```python
from build123d import *

# Parameters (mm, degrees)
LINEAR_AUSTRAGEN1_DEPTH      = 31.8
SKIZZE2_W                    = 3
SKIZZE2_H                    = 2
LINEAR_AUSTRAGEN2_DEPTH      = 2
SKIZZE4_W                    = 150
SKIZZE4_H                    = 1.45
LINEAR_START                 = -18
LINEAR_AUSTRAGEN3_DEPTH      = 18
LINEAR_AUSTRAGEN4_DEPTH      = 18
LINEAR_AUSTRAGEN5_DEPTH      = 0.5
LINEAR_AUSTRAGEN5_DEPTH_BACK = 0.5
SKIZZE8_W                    = 1
SKIZZE8_H                    = 2
LINEAR_AUSTRAGEN6_DEPTH      = 2.6
LINEAR_START_2               = -2.1
LINEAR_AUSTRAGEN7_DEPTH      = 2.1


with BuildPart() as part:
    # Skizze1 → Linear austragen1 (new body)
    with BuildSketch(Plane.XY):
        with BuildLine():
            Line((-2.5, -2.1), (2.5, -2.1))
            Line((2.5, -2.1), (2.5, 2))
            ThreePointArc((2.5, 2), (0, 2.5), (-2.5, 2))
            Line((-2.5, 2), (-2.5, -2.1))
        make_face()
    extrude(amount=LINEAR_AUSTRAGEN1_DEPTH)

    # Skizze2 → Rotation1 (revolve)
    with BuildSketch(Plane(origin=(0, 0, 0), x_dir=(0, 0, -1), z_dir=(1, 0, 0)), mode=Mode.PRIVATE) as rotation1_sk:
        with Locations((1.5, 1)):
            Rectangle(SKIZZE2_W, SKIZZE2_H)
    revolve(rotation1_sk.sketch.rotate(Axis((0, 0, -3), (0, 0, 1)), 270), axis=Axis((0, 0, -3), (0, 0, 1)))

    # Skizze3 → Linear austragen2 (add)
    with BuildSketch(Plane(origin=(0, 2.6, 0), x_dir=(-1, 0, 0), z_dir=(0, 1, 0))):
        Polygon((2.5, 23.05), (0.2, 23.05), (0.2, 24.35), (-0.2, 24.35), (-0.2, 23.05), (-2.5, 23.05), (-2.5, 22.65), (-0.2, 22.65), (-0.2, 21.35), (0.2, 21.35), (0.2, 22.65), (2.5, 22.65), align=None)
    extrude(amount=-LINEAR_AUSTRAGEN2_DEPTH)

    # Skizze4 → Rotation2 (revolve)
    with BuildSketch(Plane(origin=(0, 0, 0), x_dir=(0, 0, -1), z_dir=(1, 0, 0)), mode=Mode.PRIVATE) as rotation2_sk:
        with Locations((78, 0.725)):
            Rectangle(SKIZZE4_W, SKIZZE4_H)
    revolve(rotation2_sk.sketch.rotate(Axis((0, 0, -153), (0, 0, 1)), 270), axis=Axis((0, 0, -153), (0, 0, 1)))

    # Skizze5 → Linear austragen3 (add)
    with BuildSketch(Plane.XY.offset(-8).offset(LINEAR_START)):
        with BuildLine():
            Line((-2.95, 2.95), (-2.95, -1.95))
            Line((-2.95, -1.95), (-1.95, -2.95))
            Line((-1.95, -2.95), (1.95, -2.95))
            Line((1.95, -2.95), (2.95, -1.95))
            Line((2.95, -1.95), (2.95, 2.95))
            Line((2.95, 2.95), (1.95, 2.95))
            Line((1.95, 2.95), (1.320214964, 0.599610248))
            ThreePointArc((1.320214964, 0.599610248), (0, -1.45), (-1.320214964, 0.599610248))
            Line((-1.320214964, 0.599610248), (-1.95, 2.95))
            Line((-1.95, 2.95), (-2.95, 2.95))
        make_face()
    extrude(amount=LINEAR_AUSTRAGEN3_DEPTH)

    # Skizze6 → Linear austragen4 (add)
    with BuildSketch(Plane.XY.offset(-148)):
        with BuildLine():
            Line((-2.95, 2.95), (-2.95, -1.95))
            Line((-2.95, -1.95), (-1.95, -2.95))
            Line((-1.95, -2.95), (1.95, -2.95))
            Line((1.95, -2.95), (2.95, -1.95))
            Line((2.95, -1.95), (2.95, 2.95))
            Line((2.95, 2.95), (1.95, 2.95))
            Line((1.95, 2.95), (1.320214964, 0.599610248))
            ThreePointArc((1.320214964, 0.599610248), (0, -1.45), (-1.320214964, 0.599610248))
            Line((-1.320214964, 0.599610248), (-1.95, 2.95))
            Line((-1.95, 2.95), (-2.95, 2.95))
        make_face()
    extrude(amount=LINEAR_AUSTRAGEN4_DEPTH)

    # Skizze7 → Rotation3 (revolve)
    with BuildSketch(Plane(origin=(0, 0, 0), x_dir=(0, 0, -1), z_dir=(1, 0, 0)), mode=Mode.PRIVATE) as rotation3_sk:
        with BuildLine():
            Line((153, 0), (153, 2.5))
            Line((153, 2.5), (153.5, 3))
            Line((153.5, 3), (154, 3))
            ThreePointArc((154, 3), (154.75, 2.799038106), (155.5, 3))
            Line((155.5, 3), (156, 3))
            ThreePointArc((156, 3), (156.5, 2.866025404), (157, 3))
            Line((157, 3), (162.82871818, 3))
            Line((162.82871818, 3), (168.5, 4))
            Line((168.5, 4), (178.5, 4))
            Line((178.5, 4), (178.5, 3.5))
            Line((178.5, 3.5), (179.5, 3.5))
            Line((179.5, 3.5), (179.5, 4))
            Line((179.5, 4), (179.8, 4.3))
            Line((179.8, 4.3), (180.2, 4.3))
            Line((180.2, 4.3), (180.7, 4.8))
            Line((180.7, 4.8), (185.5, 4.8))
            Line((185.5, 4.8), (186, 4.3))
            Line((186, 4.3), (186, 4))
            Line((186, 4), (192.3865, 4))
            Line((192.3865, 4), (193, 3.3865))
            Line((193, 3.3865), (194, 3.3865))
            Line((194, 3.3865), (194, 0))
            Line((194, 0), (153, 0))
        make_face()
    revolve(rotation3_sk.sketch.rotate(Axis((0, 0, -194), (0, 0, 1)), 270), axis=Axis((0, 0, -194), (0, 0, 1)))

    # Skizze8 → Linear austragen5 (cut, two sides: drawn at the far end of the back side and taken through both)
    with BuildSketch(Plane(origin=(0, 2.6, 0), x_dir=(-1, 0, 0), z_dir=(0, 1, 0)).offset(-LINEAR_AUSTRAGEN5_DEPTH_BACK)):
        with Locations((1.5, 27)):
            Rectangle(SKIZZE8_W, SKIZZE8_H)
    extrude(amount=LINEAR_AUSTRAGEN5_DEPTH + LINEAR_AUSTRAGEN5_DEPTH_BACK, mode=Mode.SUBTRACT)

    # Skizze9 → Linear austragen6 (cut)
    with BuildSketch(Plane(origin=(0, 2.6, 0), x_dir=(-1, 0, 0), z_dir=(0, 1, 0))):
        with BuildLine():
            Line((5, 8), (5, 12.5))
            Line((5, 12.5), (1.302881422, 12.5))
            ThreePointArc((1.302881422, 12.5), (0, 12.85), (-1.302881422, 12.5))
            Line((-1.302881422, 12.5), (-5, 12.5))
            Line((-5, 12.5), (-5, 8))
            Line((-5, 8), (-1.302881422, 8))
            ThreePointArc((-1.302881422, 8), (0, 7.65), (1.302881422, 8))
            Line((1.302881422, 8), (5, 8))
        make_face()
    extrude(amount=-LINEAR_AUSTRAGEN6_DEPTH, mode=Mode.SUBTRACT)

    # Skizze10 → Rotation4 (revolve)
    with BuildSketch(Plane(origin=(0, 0, 0), x_dir=(0, 0, -1), z_dir=(1, 0, 0)), mode=Mode.PRIVATE) as rotation4_sk:
        with BuildLine():
            Line((-10.25, 2), (-8.25, 2))
            ThreePointArc((-8.25, 2), (-7.896446609, 1.853553391), (-7.75, 1.5))
            Line((-7.75, 1.5), (-7.75, 0))
            Line((-7.75, 0), (-10.25, 0))
            Line((-10.25, 0), (-10.25, 2))
        make_face()
    revolve(rotation4_sk.sketch.rotate(Axis((0, 0, 10.25), (0, 1, 0)), 180), axis=Axis((0, 0, 10.25), (0, 1, 0)))

    # Skizze11 → Linear austragen7 (cut)
    with BuildSketch(Plane(origin=(0, 2.6, 0), x_dir=(-1, 0, 0), z_dir=(0, 1, 0)).offset(LINEAR_START_2)):
        with BuildLine():
            Line((0.866025404, 10.25), (0.433012702, 11))
            Line((0.433012702, 11), (0.25, 11))
            Line((0.25, 11), (0.25, 12.737468593))
            ThreePointArc((0.25, 12.737468593), (0, 12.75), (-0.25, 12.737468593))
            Line((-0.25, 12.737468593), (-0.25, 11))
            Line((-0.25, 11), (-0.433012702, 11))
            Line((-0.433012702, 11), (-0.866025404, 10.25))
            Line((-0.866025404, 10.25), (-0.433012702, 9.5))
            Line((-0.433012702, 9.5), (-0.25, 9.5))
            Line((-0.25, 9.5), (-0.25, 7.762531407))
            ThreePointArc((-0.25, 7.762531407), (0, 7.75), (0.25, 7.762531407))
            Line((0.25, 7.762531407), (0.25, 9.5))
            Line((0.25, 9.5), (0.433012702, 9.5))
            Line((0.433012702, 9.5), (0.866025404, 10.25))
        make_face()
    extrude(amount=LINEAR_AUSTRAGEN7_DEPTH, mode=Mode.SUBTRACT)


solid = part.part
```
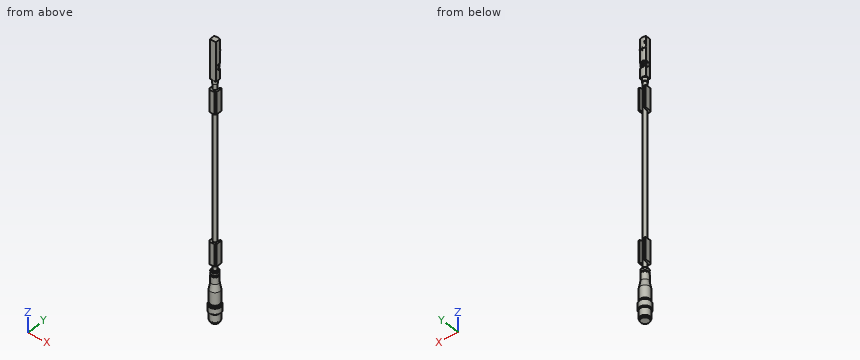
The listing builds one solid part. Answer for the finished solid, in the listing's coordinates (mm). Coordinates: 2 decimals unless noted, no trailing zeros. Order: outer loops, then holes, each group sorted by start corner. A loop starts at its lowest first (then second) coordinate and runs counter-clockwise, first axis right, second up. Notation, with made-up numbers: M 25.25,18.5 L 59.25,18.5 A7 cw 59.25,26.5 Z; hole C 9,-35 d5. An arc over 180 degrees is marked long. Answer as a JSON object with one key per item and string values. Group by question number.
1. Section A-A on z = -13.5 is taken. Write down the section's boundary in (x, y), then the cut area to 3 significant figures.
2. Flat-ended cylindrical pins translate along their axes: P1, Ø3, axis at y = -2.5, z = -86, coming from the -X side; P2, Ø3, axis at x = -0.5, z = -146.5, coming from the +Y side; P3, Ø3, axis at x = 0, z = -98.5, coming from the -Y side. Find the tip coordinate at first contact, or state that the pin passes through.
3. Straight lines are drawn through the part: line 1 (Z direction, x = 0.75, y = -1.5); line 2 (Z direction, x = -1.5, y = -2); line 3 (Y direction, x = 0.25, z = -94.5). For each, find the intervals that lie inside material, in ascending order.
4. Section B-B on z = -56.5 is taken. Write down the section's boundary in (x, y).
Values follow:
{
 "1": {"outline": "M -2.95,-1.95 L -1.95,-2.95 L 1.95,-2.95 L 2.95,-1.95 L 2.95,2.95 L 1.95,2.95 L 1.32,0.6 A1.45 ccw -1.32,0.6 L -1.95,2.95 L -2.95,2.95 Z", "area": "27.7 mm2"},
 "2": {"P1": "x = -1.05", "P2": "y = 2.95", "P3": "y = -1.45"},
 "3": {"line 1": "-194 to -153, -148 to -130, -26 to -8, -3 to 31.8", "line 2": "-194 to -153, -148 to -130, -26 to -8, 0 to 31.8", "line 3": "-1.43 to 1.43"},
 "4": {"outline": "C 0,0 d2.9"}
}
